Source: CAD feature listing. Evaluate the final solid. Frame: model axes, mm. A direction names the side the tool comes from. Give positions to 0.01 mm unless a question says otherwise; leave off trailing zeros. Loops run counter-clockwise (first coordinate to the right, second up) from the corner with the lowest first, then second, coordinate; pieces in that order, holes last.
from build123d import *

# Parameters (mm, degrees)
SKETCH1_W                = 40.5
SKETCH1_H                = 20.3
BOSS_EXTRUDE1_DEPTH      = 37.4
SKETCH2_R                = 7
BOSS_EXTRUDE2_DEPTH      = 2
CHAMFER1_SIZE            = 2
SKETCH3_R                = 3
SKETCH3_R_2              = 1.1
BOSS_EXTRUDE3_DEPTH      = 3.8
SKETCH4_W                = 8
SKETCH4_H                = 18.3
BOSS_EXTRUDE4_DEPTH      = 2.5
CUT_EXTRUDE1_DEPTH       = 43.01719886
BOSS_EXTRUDE5_DEPTH      = 1
MIRROR3_COPY_1_DEPTH     = 43.01719886
FILLET2_R                = 1.5
SKETCH7_W                = 7.5
SKETCH7_H                = 4
BOSS_EXTRUDE6_DEPTH      = 5
BOSS_EXTRUDE7_DEPTH      = 5
DRAFT1_ANGLE             = 5
FILLET3_R                = 1.5
CUT_EXTRUDE2_DEPTH       = 2
CHAMFER2_SIZE            = 1
CHAMFER2_OF_MIRROR4_SIZE = 1
MIRROR5_START            = 18.75
MIRROR5_3_DEPTH          = 2.25
MIRROR5_START_2          = -11
MIRROR5_4_DEPTH          = 2.35
MIRROR5_START_3          = 8.65
MIRROR5_5_DEPTH          = 2.35
SKETCH10_W               = 40.5
SKETCH10_H               = 20.3
CUT_EXTRUDE3_DEPTH       = 1
CUT_EXTRUDE4_DEPTH       = 1


with BuildPart() as part:
    # Sketch1 → Boss-Extrude1 (new body)
    with BuildSketch(Plane(origin=(0, 0, 0), x_dir=(1, 0, 0), z_dir=(0, 1, 0))):
        Rectangle(SKETCH1_W, SKETCH1_H)
    extrude(amount=BOSS_EXTRUDE1_DEPTH)

    # Sketch2 → Boss-Extrude2 (add)
    with BuildSketch(Plane(origin=(0, 37.4, 0), x_dir=(1, 0, 0), z_dir=(0, 1, 0))):
        with Locations(Location((-10.1, 0, 0), (0, 0, 270))):
            Circle(SKETCH2_R)
    extrude(amount=BOSS_EXTRUDE2_DEPTH)

    # Chamfer1
    chamfer1_edges = [part.edges().sort_by_distance(p)[0] for p in [
        (-10.1, 39.4, -7),
    ]]
    chamfer(chamfer1_edges, length=CHAMFER1_SIZE - 0.0001)  # a hair under: the kernel refuses the full size

    # Sketch3 → Boss-Extrude3 (add)
    with BuildSketch(Plane(origin=(0, 39.4, 0), x_dir=(1, 0, 0), z_dir=(0, 1, 0))):
        with Locations(Location((-10.1, 0, 0), (0, 0, 90))):
            Circle(SKETCH3_R)
        with Locations(Location((-10.1, 0, 0), (0, 0, 90))):
            Circle(SKETCH3_R_2, mode=Mode.SUBTRACT)
    extrude(amount=BOSS_EXTRUDE3_DEPTH)

    # Sketch4 → Boss-Extrude4 (add)
    with BuildSketch(Plane(origin=(0, 29.4, 0), x_dir=(1, 0, 0), z_dir=(0, 1, 0))):
        with Locations((-24.25, 0)):
            Rectangle(SKETCH4_W, SKETCH4_H)
    boss_extrude4 = extrude(amount=-BOSS_EXTRUDE4_DEPTH)

    # Sketch5 → Cut-Extrude1 (cut, through all)
    with BuildSketch(Plane(origin=(0, 29.4, 0), x_dir=(1, 0, 0), z_dir=(0, 1, 0))):
        with BuildLine():
            Line((-25.45, -3.2), (-23.05, -3.2))
            ThreePointArc((-23.05, -3.2), (-21.25, -5), (-23.05, -6.8))
            Line((-23.05, -6.8), (-25.45, -6.8))
            ThreePointArc((-25.45, -6.8), (-26.35, -6.558845727), (-27.008845727, -5.9))
            Line((-27.008845727, -5.9), (-28.25, -5.9))
            Line((-28.25, -5.9), (-28.25, -4.1))
            Line((-28.25, -4.1), (-27.008845727, -4.1))
            ThreePointArc((-27.008845727, -4.1), (-26.35, -3.441154273), (-25.45, -3.2))
        make_face()
    cut_extrude1 = extrude(amount=-CUT_EXTRUDE1_DEPTH, mode=Mode.SUBTRACT)

    # Mirror2: Cut-Extrude1 across plane
    add(cut_extrude1.mirror(Plane.XY), mode=Mode.SUBTRACT)

    # Sketch6 → Boss-Extrude5 (add, symmetric)
    with BuildSketch(Plane.XY):
        Polygon((-28.25, 29.4), (-20.25, 29.4), (-20.25, 31.4), align=None)
    boss_extrude5 = extrude(amount=BOSS_EXTRUDE5_DEPTH, both=True)

    # Mirror3: Boss-Extrude4, Cut-Extrude1, Boss-Extrude5 across plane
    add(boss_extrude4.mirror(Plane(origin=(0, 0, 0), x_dir=(0, 0, 1), z_dir=(1, 0, 0))))
    add(cut_extrude1.mirror(Plane(origin=(0, 0, 0), x_dir=(0, 0, 1), z_dir=(1, 0, 0))), mode=Mode.SUBTRACT)
    add(boss_extrude5.mirror(Plane(origin=(0, 0, 0), x_dir=(0, 0, 1), z_dir=(1, 0, 0))))

    # Mirror3 copy 1 sketch → Mirror3 copy 1 (cut, through all)
    with BuildSketch(Plane(origin=(0, 29.4, 0), x_dir=(-1, 0, 0), z_dir=(0, 1, 0))):
        with BuildLine():
            Line((-25.45, -3.2), (-23.05, -3.2))
            ThreePointArc((-23.05, -3.2), (-21.25, -5), (-23.05, -6.8))
            Line((-23.05, -6.8), (-25.45, -6.8))
            ThreePointArc((-25.45, -6.8), (-26.35, -6.558845727), (-27.008845727, -5.9))
            Line((-27.008845727, -5.9), (-28.25, -5.9))
            Line((-28.25, -5.9), (-28.25, -4.1))
            Line((-28.25, -4.1), (-27.008845727, -4.1))
            ThreePointArc((-27.008845727, -4.1), (-26.35, -3.441154273), (-25.45, -3.2))
        make_face()
    extrude(amount=-MIRROR3_COPY_1_DEPTH, mode=Mode.SUBTRACT)

    # Fillet2
    fillet2_edges = [part.edges().sort_by_distance(p)[0] for p in [
        (28.25, 28.15, -9.15),
        (28.25, 28.15, 9.15),
        (-28.25, 28.15, 9.15),
        (-28.25, 28.15, -9.15),
    ]]
    fillet(fillet2_edges, radius=FILLET2_R)

    # Sketch7 → Boss-Extrude6 (add)
    with BuildSketch(Plane.ZY.offset(20.25)):
        with Locations((0, 3)):
            Rectangle(SKETCH7_W, SKETCH7_H)
    extrude(amount=BOSS_EXTRUDE6_DEPTH)

    # Sketch8 → Boss-Extrude7 (add)
    with BuildSketch(Plane.ZY.offset(25.25)):
        with BuildLine():
            ThreePointArc((-0.65, 3.259807621), (-2, 3), (-0.65, 2.740192379))
            ThreePointArc((-0.65, 2.740192379), (0, 2.3), (0.65, 2.740192379))
            ThreePointArc((0.65, 2.740192379), (2, 3), (0.65, 3.259807621))
            ThreePointArc((0.65, 3.259807621), (0, 3.7), (-0.65, 3.259807621))
        make_face()
    extrude(amount=BOSS_EXTRUDE7_DEPTH)

    # Draft1
    draft1_faces = [part.faces().sort_by_distance(p)[0] for p in [
        (-22.75, 1, 0),
        (-22.75, 3, -3.75),
        (-22.75, 3, 3.75),
        (-22.75, 5, 0),
    ]]
    draft(draft1_faces, Plane(origin=(-20.25, 37.4, -10.15), x_dir=(0, 0, -1), z_dir=(-1, 0, 0)), DRAFT1_ANGLE)

    # Fillet3
    fillet3_edges = [part.edges().sort_by_distance(p)[0] for p in [
        (-22.75, 4.781278341, -3.531278341),
        (-22.75, 1.218721659, -3.531278341),
        (-22.75, 1.218721659, 3.531278341),
        (-22.75, 4.781278341, 3.531278341),
    ]]
    fillet(fillet3_edges, radius=FILLET3_R)

    # Sketch9 → Cut-Extrude2 (cut)
    with BuildSketch(Plane.XZ):
        with BuildLine():
            Line((-20.25, 10.15), (-20.25, 5.65))
            Line((-20.25, 5.65), (-18.75, 5.65))
            ThreePointArc((-18.75, 5.65), (-16.628679656, 6.528679656), (-15.75, 8.65))
            Line((-15.75, 8.65), (-15.75, 10.15))
            Line((-15.75, 10.15), (-20.25, 10.15))
        make_face()
    cut_extrude2 = extrude(amount=-CUT_EXTRUDE2_DEPTH, mode=Mode.SUBTRACT)

    # Chamfer2
    chamfer2_edges = [part.edges().sort_by_distance(p)[0] for p in [
        (-19.5, 0, 5.65),
        (-16.628679656, 0, 6.528679656),
        (-15.75, 0, 9.4),
    ]]
    chamfer(chamfer2_edges, length=CHAMFER2_SIZE)

    # Mirror4: Cut-Extrude2 across plane
    add(cut_extrude2.mirror(Plane.XY), mode=Mode.SUBTRACT)

    # Chamfer2 of Mirror4
    chamfer2_of_mirror4_edges = [part.edges().sort_by_distance(p)[0] for p in [
        (-19.5, 0, -5.65),
        (-16.628679656, 0, -6.528679656),
        (-15.75, 0, -9.4),
    ]]
    chamfer(chamfer2_of_mirror4_edges, length=CHAMFER2_OF_MIRROR4_SIZE)

    # Mirror5: read off the stored shape, not the designer's step
    # Mirror5 outline → Mirror5 (revolve, cut)
    with BuildSketch(Plane(origin=(18.75, 0, -8.65), x_dir=(1, 0, 0), z_dir=(0, 0, 1))):
        Polygon((3, 1), (3, 2), (0, 2), (0, 0), (4, 0), align=None)
    revolve(axis=Axis((18.75, 0, -8.65), (0, 1, 0)), mode=Mode.SUBTRACT)

    # Mirror5 2 outline → Mirror5 2 (revolve, cut)
    with BuildSketch(Plane(origin=(18.75, 0, 8.65), x_dir=(1, 0, 0), z_dir=(0, 0, 1))):
        Polygon((3, 1), (3, 2), (0, 2), (0, 0), (4, 0), align=None)
    revolve(axis=Axis((18.75, 0, 8.65), (0, 1, 0)), mode=Mode.SUBTRACT)

    # Mirror5 3 outline → Mirror5 3 (cut)
    with BuildSketch(Plane.YZ.offset(MIRROR5_START)):
        Polygon((1, -5.65), (0, -4.65), (0, -10.15), (2, -10.15), (2, -5.65), align=None)
        Polygon((1, 5.65), (2, 5.65), (2, 10.15), (0, 10.15), (0, 4.65), align=None)
    extrude(amount=MIRROR5_3_DEPTH, mode=Mode.SUBTRACT)

    # Mirror5 4 outline → Mirror5 4 (cut)
    with BuildSketch(Plane.XY.offset(MIRROR5_START_2)):
        Polygon((15.75, 2), (15.75, 1), (14.75, 0), (20.25, 0), (20.25, 2), align=None)
    extrude(amount=MIRROR5_4_DEPTH, mode=Mode.SUBTRACT)

    # Mirror5 5 outline → Mirror5 5 (cut)
    with BuildSketch(Plane.XY.offset(MIRROR5_START_3)):
        Polygon((15.75, 2), (15.75, 1), (14.75, 0), (20.25, 0), (20.25, 2), align=None)
    extrude(amount=MIRROR5_5_DEPTH, mode=Mode.SUBTRACT)

    # Sketch10 → Cut-Extrude3 (cut)
    with BuildSketch(Plane(origin=(0, 37.4, 0), x_dir=(1, 0, 0), z_dir=(0, 1, 0))):
        Rectangle(SKETCH10_W, SKETCH10_H)
        Polygon((-18.1, -8), (14.25, -8), (15.75, 0), (14.25, 8), (-18.1, 8), align=None, mode=Mode.SUBTRACT)
    extrude(amount=-CUT_EXTRUDE3_DEPTH, mode=Mode.SUBTRACT)

    # Sketch11 → Cut-Extrude4 (cut)
    with BuildSketch(Plane(origin=(0, 36.4, 0), x_dir=(1, 0, 0), z_dir=(0, 1, 0))):
        with BuildLine():
            Line((16.842885351, 2.310688429), (16.10573121, 6.242177176))
            ThreePointArc((16.10573121, 6.242177176), (16.904314862, 7.409337898), (18.071475584, 6.610754247))
            Line((18.071475584, 6.610754247), (18.808629724, 2.679265499))
            ThreePointArc((18.808629724, 2.679265499), (18.010046072, 1.512104777), (16.842885351, 2.310688429))
        make_face()
    cut_extrude4 = extrude(amount=-CUT_EXTRUDE4_DEPTH, mode=Mode.SUBTRACT)

    # Mirror6: Cut-Extrude4 across plane
    add(cut_extrude4.mirror(Plane.XY), mode=Mode.SUBTRACT)


solid = part.part
1) Cut plane B-B (y = 34.5). Return loops of the section in (x, z), and give its area (3 significant figures).
Checks:
outline: (-20.25, -10.15) - (20.25, -10.15) - (20.25, 10.15) - (-20.25, 10.15) - close
area: 822 mm2
2) Pull-direction query (Z, two-part tool) for faces 1 (the cylindrical face through (-21.25, 28.17, 4.96)), 2 (the cylindrical face through (-22.8, 4.33, 3.1)), 3 (the flat face through (2, 37.4, 0)); classes: released by +Z, released by -Z, zero draft, split by the parting line, or undercut.
Checks:
face 1: undercut
face 2: released by +Z
face 3: zero draft
3) Cut plane C-C (x = 6). Return loops of the section in (y, z), and give its area (3 significant figures).
Checks:
outline: (0, -10.15) - (36.4, -10.15) - (36.4, -8) - (37.4, -8) - (37.4, 8) - (36.4, 8) - (36.4, 10.15) - (0, 10.15) - close
area: 755 mm2
4) Contact query for flat-ended pins moving along their axis: P1, Ø1.2, axis at x = 24, y = 28, coming from the -Z side; P2, Ø1, axis at x = -27.5, y = 28.5, coming from the -Z side; P3, Ø10, axis at y = 14.5, z = 3, coming from the -X side. Output: stop coordinate, or through.
Checks:
P1: stops at z = -9.15
P2: stops at z = -9.13
P3: stops at x = -20.25
5) Reachability of faces 4 (the flat face through (18, 2, -8)), 5 (the flat face through (28, 28, -5.9)), 6 (the cylindrical face through (21.25, 28.17, 4.96)) from +Z, -Z, +X, -X, +Y, -Y: full face, straight path, thin tool, end or side. Return the list, or none.
Checks:
face 4: -Z, +X, -Y
face 5: +X, +Y, -Y
face 6: +Y, -Y
6) Ray query, probe 1 along Z at (x, y) = (-10, 41); probe 2 along X at (y, z) = (40.5, 0); probe 3 along Y at (x, z) = (4, -4). Return the intervals inside material, ascending.
Checks:
probe 1: z = -3 to -1.1, 1.1 to 3
probe 2: x = -13.1 to -11.2, -9 to -7.1
probe 3: y = 0 to 37.4
